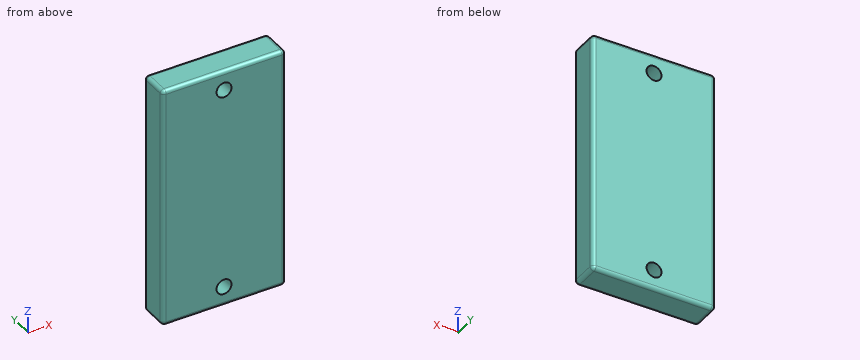
from build123d import *

# Parameters (mm, degrees)
CROQUIS1_W              = 33
CROQUIS1_H              = 65
SALIENTE_EXTRUIR1_DEPTH = 8
REDONDEO1_R             = 1
CROQUIS2_R              = 2
CORTAR_EXTRUIR1_DEPTH   = 74.334848469


with BuildPart() as part:
    # Croquis1 → Saliente-Extruir1 (new body)
    with BuildSketch(Plane(origin=(0, 0, 0), x_dir=(1, 0, 0), z_dir=(0, 1, 0))):
        with Locations((16.5, 32.5)):
            Rectangle(CROQUIS1_W, CROQUIS1_H)
    extrude(amount=SALIENTE_EXTRUIR1_DEPTH)

    # Redondeo1
    redondeo1_edges = [part.edges().sort_by_distance(p)[0] for p in [
        (33, 8, -32.5),
        (16.5, 8, -65),
        (0, 8, -32.5),
        (16.5, 0, -65),
        (33, 0, -32.5),
        (16.5, 0, 0),
        (0, 0, -32.5),
        (16.5, 8, 0),
        (0, 4, -65),
        (33, 4, -65),
        (33, 4, 0),
        (0, 4, 0),
    ]]
    fillet(redondeo1_edges, radius=REDONDEO1_R)

    # Croquis2 → Cortar-Extruir1 (cut, through all)
    with BuildSketch(Plane(origin=(0, 8, 0), x_dir=(1, 0, 0), z_dir=(0, 1, 0))):
        with Locations(Location((16.5, 5.25, 0), (0, 0, 270))):
            Circle(CROQUIS2_R)
        with Locations(Location((16.5, 59.75, 0), (0, 0, 270))):
            Circle(CROQUIS2_R)
    extrude(amount=-CORTAR_EXTRUIR1_DEPTH, mode=Mode.SUBTRACT)


solid = part.part
Verification items for the finished model (mm, model axes). Coordinates: 2 decimals unless noted, no trailing zeros. Order: outer loops, then holes, each group sorted by start corner. A loop starts at its lowest first (then second) coordinate and runs counter-clockwise, first axis right, second up.
Item 1: Section check B-B, the plane x = 16.5. Enter the section's corners in (y, z).
Filled in:
outline: (0, -64) arc R1 ccw to (1, -65) - (7, -65) arc R1 ccw to (8, -64) - (8, -61.75) - (0, -61.75) - close; (0, -57.75) - (8, -57.75) - (8, -7.25) - (0, -7.25) - close; (0, -3.25) - (8, -3.25) - (8, -1) arc R1 ccw to (7, 0) - (1, 0) arc R1 ccw to (0, -1) - close
Item 2: Material ranges on L1, parallel to X at y = 2.5, z = -59.75; L2, parallel to Z at x = 18, y = 5; L3, parallel to Z at x = 31.5, y = 7.75, recorded low to high.
Filled in:
L1: x = 0 to 14.5, 18.5 to 33
L2: z = -65 to -61.07, -58.43 to -6.57, -3.93 to 0
L3: z = -64.66 to -0.34
Item 3: Section check C-C, the plane z = -6.5. Enter the section's corners in (x, y), then the cut area to 3 significant figures.
Filled in:
outline: (0, 1) arc R1 ccw to (1, 0) - (14.94, 0) - (14.94, 8) - (1, 8) arc R1 ccw to (0, 7) - close; (18.06, 0) - (32, 0) arc R1 ccw to (33, 1) - (33, 7) arc R1 ccw to (32, 8) - (18.06, 8) - close
area: 238 mm2
Item 4: Section check A-A, the plane z = -59. Enter the section's corners in (x, y).
Filled in:
outline: (0, 1) arc R1 ccw to (1, 0) - (14.65, 0) - (14.65, 8) - (1, 8) arc R1 ccw to (0, 7) - close; (18.35, 0) - (32, 0) arc R1 ccw to (33, 1) - (33, 7) arc R1 ccw to (32, 8) - (18.35, 8) - close
Item 5: Depth check by flat-ended pin: pin 1 (3.5 mm diameter, centred on x = 16.5, z = -59.75, fed in from +Y). Enter the tip coordinate at first touch or a pass-through.
Filled in:
pin 1: passes through
